Geometry: final body of the model. Coordinates: model frame, mm. A direction names the side the tool comes from. Give positions to 0.01 mm unless a question says otherwise; leave off trailing zeros. Write each loop counter-clockwise with the first axis right and the second up, starting at its lowest first coordinate (ties: lowest second). Pieces come first, ordered by that corner, then holes. Notation, with made-up numbers: M 8,-29 L 44,-29 A19 ccw 44,-4 Z; hole C 17,73.25 d1. An arc over 180 degrees is marked long. Use a Markdown table: item, result. Add a question column.
1) Line query: line 1 (Y direction, x = 4, z = 4.5); line 2 (Z direction, x = -19, y = 27.5); line 3 (Z direction, x = -6, y = -9). Output: solid intervals per line, ascending.
2) Section D-D on x = -6.5. Return the cut outline in (y, z).
3) Section C-C on x = -14.5. Return the cut outline in (y, z), then the cut area to 3 significant figures.
4) Section A-A on z = 31. Return the cut outline in (x, y), then the cut area to 3 significant figures.
5) Set-up query: faces 1 (the flat face through (-10, 15, 17)), 2 (the flat face through (-4, -2, 28)), 3 (the flat face through (-4, 14, 17)), 4 (the flat face through (-15, 0, 4)), 5 (the cylindrical face through (-2.797, -9.141, 17.198)). Return all of +Z, -Z, +X, -X, +Y, -Y with unobstructed straight access to the full face (end or side cutting, diameter ignored); none if empty.
6) Section B-B on y = 0. State how many separate pieces and enclosed holes the cut face has, then the cut area to 3 significant figures.
7) Pin query (flat end, axial travel): pin 1 (10 mm diameter, centred on y = -14, z = 35, fed in from +X); pin 2 (8 mm diameter, centred on x = 0.5, y = 19, fed in from +Z); pin 3 (2 mm diameter, centred on y = 7.5, z = 8.5, fed in from -X); pin 4 (8 mm diameter, centred on x = 12.5, y = 10.5, fed in from +Z). Return the tip coordinate at first contact, or that it passes through.
8) Draft query along Z for faces 6 (the cylindrical face through (0.056, -6.859, 39.797)), 7 (the cylindrical face through (10.82, 15.06, 1.97)), 8 (the cylindrical face through (-8.37, -11.21, 5.19)). Return one class per face: +Z half, -Z half, draft (parallel to the pull), parting line (faces both ways), or undercut.
```python
from build123d import *

# Parameters (mm, degrees)
SKETCH1_R           = 35
SKETCH1_R_2         = 3
BOSS_EXTRUDE1_DEPTH = 6
SKETCH4_R           = 5
CUT_EXTRUDE1_DEPTH  = 2
SKETCH5_W           = 8
SKETCH5_H           = 16
BOSS_EXTRUDE2_DEPTH = 35
SKETCH6_R           = 3.25
CUT_EXTRUDE2_DEPTH  = 67.535704701
FILLET1_R           = 8
FILLET2_R           = 4
SKETCH7_W           = 6
SKETCH7_H           = 30
BOSS_EXTRUDE3_DEPTH = 12
FILLET3_R           = 4


with BuildPart() as part:
    # Sketch1 → Boss-Extrude1 (new body)
    with BuildSketch(Plane.XY):
        Circle(SKETCH1_R)
        with Locations((0, 18.425417274)):
            Circle(SKETCH1_R_2, mode=Mode.SUBTRACT)
        with Locations((13.028737501, 13.028737501)):
            Circle(SKETCH1_R_2, mode=Mode.SUBTRACT)
        with Locations((18.425417274, 0)):
            Circle(SKETCH1_R_2, mode=Mode.SUBTRACT)
        with Locations((13.028737501, -13.028737501)):
            Circle(SKETCH1_R_2, mode=Mode.SUBTRACT)
        with Locations((0, -18.425417274)):
            Circle(SKETCH1_R_2, mode=Mode.SUBTRACT)
        with Locations((-13.028737501, -13.028737501)):
            Circle(SKETCH1_R_2, mode=Mode.SUBTRACT)
        with Locations((-18.425417274, 0)):
            Circle(SKETCH1_R_2, mode=Mode.SUBTRACT)
        with Locations((-13.028737501, 13.028737501)):
            Circle(SKETCH1_R_2, mode=Mode.SUBTRACT)
    extrude(amount=BOSS_EXTRUDE1_DEPTH)

    # Sketch4 → Cut-Extrude1 (cut)
    with BuildSketch(Plane.XY.offset(6)):
        with Locations((0, 18.425417274)):
            Circle(SKETCH4_R)
        with Locations((13.028737501, 13.028737501)):
            Circle(SKETCH4_R)
        with Locations((18.425417274, 0)):
            Circle(SKETCH4_R)
        with Locations((13.028737501, -13.028737501)):
            Circle(SKETCH4_R)
        with Locations((0, -18.425417274)):
            Circle(SKETCH4_R)
        with Locations((-13.028737501, -13.028737501)):
            Circle(SKETCH4_R)
        with Locations((-18.425417274, 0)):
            Circle(SKETCH4_R)
        with Locations((-13.028737501, 13.028737501)):
            Circle(SKETCH4_R)
    extrude(amount=-CUT_EXTRUDE1_DEPTH, mode=Mode.SUBTRACT)

    # Sketch5 → Boss-Extrude2 (add)
    with BuildSketch(Plane.XY.offset(6)):
        Rectangle(SKETCH5_W, SKETCH5_H)
    extrude(amount=BOSS_EXTRUDE2_DEPTH)

    # Sketch6 → Cut-Extrude2 (cut, through all)
    with BuildSketch(Plane(origin=(4, 0, 0), x_dir=(0, 0, -1), z_dir=(1, 0, 0))):
        with Locations(Location((-31, 0, 0), (0, 0, 90))):
            Circle(SKETCH6_R)
    extrude(amount=-CUT_EXTRUDE2_DEPTH, mode=Mode.SUBTRACT)

    # Fillet1
    # the kernel refuses this fillet: 8 mm, written as the material it adds along each edge
    with BuildSketch(Plane(origin=(4, 8, 6), x_dir=(1, 0, 0), z_dir=(0, -1, 0)), Plane(origin=(-4, -8, 6), x_dir=(-1, 0, 0), z_dir=(0, 1, 0))) as fillet1_piece_1:
        with BuildLine():
            CenterArc((FILLET1_R, FILLET1_R), FILLET1_R, 180, 90)
            Line((0, FILLET1_R), (0, 0))
            Line((0, 0), (FILLET1_R, 0))
        make_face()
    extrude(amount=16)
    with BuildSketch(Plane(origin=(-4, 8, 6), x_dir=(0, 1, 0), z_dir=(1, 0, 0))) as fillet1_piece_2_section:
        with BuildLine():
            CenterArc((FILLET1_R, FILLET1_R), FILLET1_R, 180, 90)
            Line((0, FILLET1_R), (0, 0))
            Line((0, 0), (FILLET1_R, 0))
        make_face()
    fillet1_piece_2 = extrude(amount=8, mode=Mode.PRIVATE)
    fillet1_piece_2 = fillet1_piece_2 - Plane(origin=(0, 18.425417274, 7.870474633), x_dir=(1, 0, 0), z_dir=(0, 0, 1)) * Cylinder(5, 48, mode=Mode.PRIVATE)
    add(fillet1_piece_2)
    with BuildSketch(Plane(origin=(4, -8, 6), x_dir=(0, -1, 0), z_dir=(-1, 0, 0))) as fillet1_piece_3_section:
        with BuildLine():
            CenterArc((FILLET1_R, FILLET1_R), FILLET1_R, 180, 90)
            Line((0, FILLET1_R), (0, 0))
            Line((0, 0), (FILLET1_R, 0))
        make_face()
    fillet1_piece_3 = extrude(amount=8, mode=Mode.PRIVATE)
    fillet1_piece_3 = fillet1_piece_3 - Plane(origin=(0, -18.425417274, 7.870474633), x_dir=(1, 0, 0), z_dir=(0, 0, 1)) * Cylinder(5, 48, mode=Mode.PRIVATE)
    add(fillet1_piece_3)
    with BuildSketch(Plane(origin=(4, 28, 6), x_dir=(1, 0, 0), z_dir=(0, -1, 0))) as fillet1_piece_4a_section:
        with BuildLine():
            CenterArc((FILLET1_R, FILLET1_R), FILLET1_R, 180, 90)
            Line((0, FILLET1_R), (0, 0))
            Line((0, 0), (FILLET1_R, 0))
        make_face()
    fillet1_piece_4a = extrude(amount=36, mode=Mode.PRIVATE)
    fillet1_piece_4a = fillet1_piece_4a - Plane(origin=(0, 18.425417274, 7.7362908), x_dir=(1, 0, 0), z_dir=(0, 0, 1)) * Cylinder(5, 104, mode=Mode.PRIVATE)
    fillet1_piece_4a = fillet1_piece_4a - Plane(origin=(13.028737501, 13.028737501, 7.7362908), x_dir=(1, 0, 0), z_dir=(0, 0, 1)) * Cylinder(5, 104, mode=Mode.PRIVATE)
    fillet1_piece_4a = split(fillet1_piece_4a, bisect_by=Plane(origin=(5.823576256, 8, 7.7362908), z_dir=(0, 1, 0)), keep=Keep.TOP, mode=Mode.PRIVATE)
    with BuildSketch(Plane(origin=(-4, 8, 6), x_dir=(0, 1, 0), z_dir=(1, 0, 0))) as fillet1_piece_4b_section:
        with BuildLine():
            CenterArc((FILLET1_R, FILLET1_R), FILLET1_R, 180, 90)
            Line((0, FILLET1_R), (0, 0))
            Line((0, 0), (FILLET1_R, 0))
        make_face()
    fillet1_piece_4b = extrude(amount=28, mode=Mode.PRIVATE)
    fillet1_piece_4b = fillet1_piece_4b - Plane(origin=(0, 18.425417274, 6.213712954), x_dir=(1, 0, 0), z_dir=(0, 0, 1)) * Cylinder(5, 88, mode=Mode.PRIVATE)
    fillet1_piece_4b = fillet1_piece_4b - Plane(origin=(13.028737501, 13.028737501, 6.213712954), x_dir=(1, 0, 0), z_dir=(0, 0, 1)) * Cylinder(5, 88, mode=Mode.PRIVATE)
    fillet1_piece_4b = split(fillet1_piece_4b, bisect_by=Plane(origin=(4, 13.913670674, 6.213712954), z_dir=(1, 0, 0)), keep=Keep.TOP, mode=Mode.PRIVATE)
    fillet1_piece_4 = fillet1_piece_4a & fillet1_piece_4b
    add(fillet1_piece_4)
    with BuildSketch(Plane(origin=(24, -8, 6), x_dir=(0, -1, 0), z_dir=(-1, 0, 0))) as fillet1_piece_5a_section:
        with BuildLine():
            CenterArc((FILLET1_R, FILLET1_R), FILLET1_R, 180, 90)
            Line((0, FILLET1_R), (0, 0))
            Line((0, 0), (FILLET1_R, 0))
        make_face()
    fillet1_piece_5a = extrude(amount=28, mode=Mode.PRIVATE)
    fillet1_piece_5a = fillet1_piece_5a - Plane(origin=(0, -18.425417274, 6.213686684), x_dir=(1, 0, 0), z_dir=(0, 0, 1)) * Cylinder(5, 88, mode=Mode.PRIVATE)
    fillet1_piece_5a = fillet1_piece_5a - Plane(origin=(13.028737501, -13.028737501, 6.213686684), x_dir=(1, 0, 0), z_dir=(0, 0, 1)) * Cylinder(5, 88, mode=Mode.PRIVATE)
    fillet1_piece_5a = split(fillet1_piece_5a, bisect_by=Plane(origin=(4, -13.913663635, 6.213686684), z_dir=(1, 0, 0)), keep=Keep.TOP, mode=Mode.PRIVATE)
    with BuildSketch(Plane(origin=(4, 8, 6), x_dir=(1, 0, 0), z_dir=(0, -1, 0))) as fillet1_piece_5b_section:
        with BuildLine():
            CenterArc((FILLET1_R, FILLET1_R), FILLET1_R, 180, 90)
            Line((0, FILLET1_R), (0, 0))
            Line((0, 0), (FILLET1_R, 0))
        make_face()
    fillet1_piece_5b = extrude(amount=36, mode=Mode.PRIVATE)
    fillet1_piece_5b = fillet1_piece_5b - Plane(origin=(0, -18.425417274, 7.736290735), x_dir=(1, 0, 0), z_dir=(0, 0, 1)) * Cylinder(5, 104, mode=Mode.PRIVATE)
    fillet1_piece_5b = fillet1_piece_5b - Plane(origin=(13.028737501, -13.028737501, 7.736290735), x_dir=(1, 0, 0), z_dir=(0, 0, 1)) * Cylinder(5, 104, mode=Mode.PRIVATE)
    fillet1_piece_5b = split(fillet1_piece_5b, bisect_by=Plane(origin=(5.823577009, -8, 7.736290735), z_dir=(0, -1, 0)), keep=Keep.TOP, mode=Mode.PRIVATE)
    fillet1_piece_5 = fillet1_piece_5a & fillet1_piece_5b
    add(fillet1_piece_5)
    with BuildSketch(Plane(origin=(-4, -8, 6), x_dir=(-1, 0, 0), z_dir=(0, 1, 0))) as fillet1_piece_6a_section:
        with BuildLine():
            CenterArc((FILLET1_R, FILLET1_R), FILLET1_R, 180, 90)
            Line((0, FILLET1_R), (0, 0))
            Line((0, 0), (FILLET1_R, 0))
        make_face()
    fillet1_piece_6a = extrude(amount=36, mode=Mode.PRIVATE)
    fillet1_piece_6a = fillet1_piece_6a - Plane(origin=(-13.028737501, 13.028737501, 7.736291892), x_dir=(1, 0, 0), z_dir=(0, 0, 1)) * Cylinder(5, 104, mode=Mode.PRIVATE)
    fillet1_piece_6a = fillet1_piece_6a - Plane(origin=(0, 18.425417274, 7.736291892), x_dir=(1, 0, 0), z_dir=(0, 0, 1)) * Cylinder(5, 104, mode=Mode.PRIVATE)
    fillet1_piece_6a = split(fillet1_piece_6a, bisect_by=Plane(origin=(-5.823575173, 8, 7.736291892), z_dir=(0, 1, 0)), keep=Keep.TOP, mode=Mode.PRIVATE)
    with BuildSketch(Plane(origin=(-24, 8, 6), x_dir=(0, 1, 0), z_dir=(1, 0, 0))) as fillet1_piece_6b_section:
        with BuildLine():
            CenterArc((FILLET1_R, FILLET1_R), FILLET1_R, 180, 90)
            Line((0, FILLET1_R), (0, 0))
            Line((0, 0), (FILLET1_R, 0))
        make_face()
    fillet1_piece_6b = extrude(amount=28, mode=Mode.PRIVATE)
    fillet1_piece_6b = fillet1_piece_6b - Plane(origin=(-13.028737501, 13.028737501, 6.213714747), x_dir=(1, 0, 0), z_dir=(0, 0, 1)) * Cylinder(5, 88, mode=Mode.PRIVATE)
    fillet1_piece_6b = fillet1_piece_6b - Plane(origin=(0, 18.425417274, 6.213714747), x_dir=(1, 0, 0), z_dir=(0, 0, 1)) * Cylinder(5, 88, mode=Mode.PRIVATE)
    fillet1_piece_6b = split(fillet1_piece_6b, bisect_by=Plane(origin=(-4, 13.913671155, 6.213714747), z_dir=(-1, 0, 0)), keep=Keep.TOP, mode=Mode.PRIVATE)
    fillet1_piece_6 = fillet1_piece_6a & fillet1_piece_6b
    add(fillet1_piece_6)
    with BuildSketch(Plane(origin=(-4, -28, 6), x_dir=(-1, 0, 0), z_dir=(0, 1, 0))) as fillet1_piece_7a_section:
        with BuildLine():
            CenterArc((FILLET1_R, FILLET1_R), FILLET1_R, 180, 90)
            Line((0, FILLET1_R), (0, 0))
            Line((0, 0), (FILLET1_R, 0))
        make_face()
    fillet1_piece_7a = extrude(amount=36, mode=Mode.PRIVATE)
    fillet1_piece_7a = fillet1_piece_7a - Plane(origin=(-13.028737501, -13.028737501, 7.736291939), x_dir=(1, 0, 0), z_dir=(0, 0, 1)) * Cylinder(5, 104, mode=Mode.PRIVATE)
    fillet1_piece_7a = fillet1_piece_7a - Plane(origin=(0, -18.425417274, 7.736291939), x_dir=(1, 0, 0), z_dir=(0, 0, 1)) * Cylinder(5, 104, mode=Mode.PRIVATE)
    fillet1_piece_7a = split(fillet1_piece_7a, bisect_by=Plane(origin=(-5.823575033, -8, 7.736291939), z_dir=(0, -1, 0)), keep=Keep.TOP, mode=Mode.PRIVATE)
    with BuildSketch(Plane(origin=(4, -8, 6), x_dir=(0, -1, 0), z_dir=(-1, 0, 0))) as fillet1_piece_7b_section:
        with BuildLine():
            CenterArc((FILLET1_R, FILLET1_R), FILLET1_R, 180, 90)
            Line((0, FILLET1_R), (0, 0))
            Line((0, 0), (FILLET1_R, 0))
        make_face()
    fillet1_piece_7b = extrude(amount=28, mode=Mode.PRIVATE)
    fillet1_piece_7b = fillet1_piece_7b - Plane(origin=(-13.028737501, -13.028737501, 6.213687212), x_dir=(1, 0, 0), z_dir=(0, 0, 1)) * Cylinder(5, 88, mode=Mode.PRIVATE)
    fillet1_piece_7b = fillet1_piece_7b - Plane(origin=(0, -18.425417274, 6.213687212), x_dir=(1, 0, 0), z_dir=(0, 0, 1)) * Cylinder(5, 88, mode=Mode.PRIVATE)
    fillet1_piece_7b = split(fillet1_piece_7b, bisect_by=Plane(origin=(-4, -13.913663776, 6.213687212), z_dir=(-1, 0, 0)), keep=Keep.TOP, mode=Mode.PRIVATE)
    fillet1_piece_7 = fillet1_piece_7a & fillet1_piece_7b
    add(fillet1_piece_7)

    # Fillet2
    fillet2_edges = [part.edges().sort_by_distance(p)[0] for p in [
        (0, 8, 41),
        (0, -8, 41),
    ]]
    fillet(fillet2_edges, radius=FILLET2_R)

    # Sketch7 → Boss-Extrude3 (add)
    with BuildSketch(Plane.ZY.offset(4)):
        with Locations((17.24, 0)):
            Rectangle(SKETCH7_W, SKETCH7_H)
    extrude(amount=BOSS_EXTRUDE3_DEPTH)

    # Fillet3
    # the kernel refuses this fillet: 4 mm, written as the material it adds along each edge
    with BuildSketch(Plane(origin=(-4, -8, 14.24), x_dir=(1, 0, 0), z_dir=(0, 0, 1))) as fillet3_piece_1:
        with BuildLine():
            CenterArc((FILLET3_R, -FILLET3_R), FILLET3_R, 90, 90)
            Line((0, -FILLET3_R), (0, 0))
            Line((0, 0), (FILLET3_R, 0))
        make_face()
    extrude(amount=6)
    with BuildSketch(Plane(origin=(-4, 8, 14.24), x_dir=(1, 0, 0), z_dir=(0, 0, 1))) as fillet3_piece_2:
        with BuildLine():
            CenterArc((FILLET3_R, FILLET3_R), FILLET3_R, 180, 90)
            Line((0, FILLET3_R), (0, 0))
            Line((0, 0), (FILLET3_R, 0))
        make_face()
    extrude(amount=6)


solid = part.part
```
Found:
| question | item | result |
|---|---|---|
| 1 | line 1 | -34.77 to -21.43, -15.43 to 15.43, 21.43 to 34.77 |
| 1 | line 2 | 0 to 6 |
| 1 | line 3 | 0 to 8.71, 14.24 to 20.24 |
| 2 | outline | M -34.39,0 L 34.39,0 L 34.39,6 L 16,6 A8 cw 10.5,8.19 L -10.5,8.19 A8 cw -16,6 L -34.39,6 Z; M -15,14.24 L 15,14.24 L 15,20.24 L -15,20.24 Z |
| 3 | outline | M -31.86,0 L -15.64,0 L -15.64,4 L -17.81,4 L -17.81,6 L -31.86,6 Z; M -15,14.24 L 15,14.24 L 15,20.24 L -15,20.24 Z; M -10.41,0 L 10.41,0 L 10.41,4 L 8.25,4 L 8.25,6 L 3.1,6 L 3.1,4 L -3.1,4 L -3.1,6 L -8.25,6 L -8.25,4 L -10.41,4 Z; M 15.64,0 L 31.86,0 L 31.86,6 L 17.81,6 L 17.81,4 L 15.64,4 Z |
| 3 | area | 470 mm² |
| 4 | outline | M -4,-8 L 4,-8 L 4,-3.25 L -4,-3.25 Z; M -4,3.25 L 4,3.25 L 4,8 L -4,8 Z |
| 4 | area | 76.0 mm² |
| 5 | face 1 | +Z, +X, -X, +Y |
| 5 | face 2 | +Z, -X, +Y, -Y |
| 5 | face 3 | +Z, +X, +Y |
| 5 | face 4 | none |
| 5 | face 5 | +Z, +X, -Y |
| 6 | separate pieces | 4 |
| 6 | enclosed holes | 0 |
| 6 | area | 659 mm² |
| 7 | pin 1 | through |
| 7 | pin 2 | z = 4 |
| 7 | pin 3 | x = -7.34 |
| 7 | pin 4 | z = 6.81 |
| 8 | face 6 | +Z half |
| 8 | face 7 | draft |
| 8 | face 8 | undercut |
